Read the model definition and answer for the solid it produces. Units are mm, in the model's axes. Face numbers are marked on the shaded views. A direction names the side the tool comes from. Coordinates: 2 decimals unless noted, no trailing zeros. Write each loop counter-clockwise with the first axis right and the second up, starting at its lowest first coordinate (ties: lowest second). Pieces come first, ordered by that corner, then holes. Notation, with made-up numbers: (51, 44.5) -> (96, 44.5) arc R28 ccw to (96, 63.5) -> close; hole circle Ø11 at (17.5, -38). An arc over 180 degrees is marked (long way). Return JSON: item names as keys, results as strings.
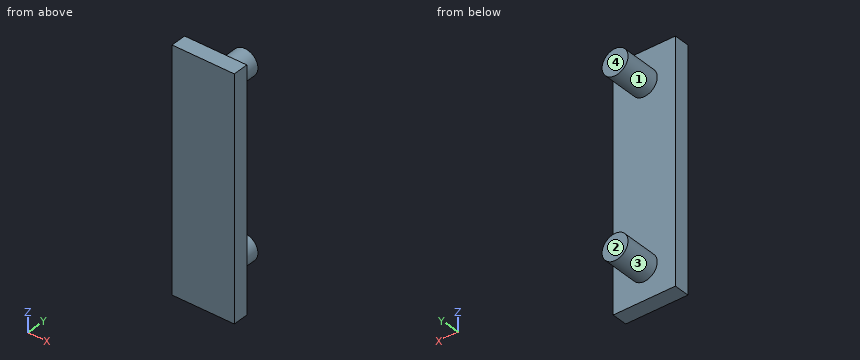
from build123d import *

# Parameters (mm, degrees)
SKETCH3_R             = 2.5
BOSS_EXTRUDE4_DEPTH   = 10
BOSS_EXTRUDE4_2_DEPTH = 10
SKETCH2_W             = 12
SKETCH2_H             = 46
BOSS_EXTRUDE5_DEPTH   = 3


with BuildPart() as part:
    # Sketch3 → Boss-Extrude4 (new body)
    with BuildSketch(Plane(origin=(0, 0, 0), x_dir=(1, 0, 0), z_dir=(0, 1, 0))):
        with Locations((-0.169934853, 17.143306367)):
            Circle(SKETCH3_R)
    extrude(amount=BOSS_EXTRUDE4_DEPTH)



with BuildPart() as body_2:
    # Sketch3 → Boss-Extrude4 2 (new body)
    with BuildSketch(Plane(origin=(0, 0, 0), x_dir=(1, 0, 0), z_dir=(0, 1, 0))):
        with Locations((-0.169934853, -16.856693633)):
            Circle(SKETCH3_R)
    extrude(amount=BOSS_EXTRUDE4_2_DEPTH)


with BuildPart() as part_1:
    add(part.part)

    add(body_2.part)  # Boss-Extrude5 merges body 2
    # Sketch2 → Boss-Extrude5 (add)
    with BuildSketch(Plane(origin=(0, 0, 0), x_dir=(1, 0, 0), z_dir=(0, 1, 0))):
        with Locations((-0.169934853, 0.143306367)):
            Rectangle(SKETCH2_W, SKETCH2_H)
    extrude(amount=BOSS_EXTRUDE5_DEPTH)


solid = part_1.part
1. A tool of negligible diameter and unlimited length cuts with its end or side. For the marked faces 1 and 2, from which of +Z, -Z, +X, -X, +Y, -Y can it reach the whole face along a straight path? Write none if from no direction.
Taken from the geometry:
{"face 1": "+Y", "face 2": "+Z, -Z, +X, -X, +Y"}
2. Consider L1, parallel to Z at x = 0, y = 4.25; L2, parallel to Y at x = 1.75, z = 9.5; L3, parallel to Z at x = 2, y = 6. Determine where each line is inside the solid, lowest interval first.
Taken from the geometry:
{"L1": "z = -19.64 to -14.65, 14.36 to 19.35", "L2": "y = 0 to 3", "L3": "z = -18.38 to -15.9, 15.62 to 18.1"}
3. The part is cut by section C-C (y = 5). Determine the outline of the cut face in (x, z).
Taken from the geometry:
{"outline": "circle Ø5 at (-0.17, -17.14); circle Ø5 at (-0.17, 16.86)"}
4. The part is cut by section A-A (x = -0.25). Determine the outline of the cut face in (y, z).
Taken from the geometry:
{"outline": "(0, -23.14) -> (3, -23.14) -> (3, -19.64) -> (10, -19.64) -> (10, -14.64) -> (3, -14.64) -> (3, 14.36) -> (10, 14.36) -> (10, 19.36) -> (3, 19.36) -> (3, 22.86) -> (0, 22.86) -> close"}
5. The part is cut by section D-D (z = -12.5). Determine the outline of the cut face in (x, y), then the cut area to 3 significant figures.
Taken from the geometry:
{"outline": "(-6.17, 0) -> (5.83, 0) -> (5.83, 3) -> (-6.17, 3) -> close", "area": "36.0 mm2"}
6. The part is cut by section B-B (z = -18). Determine the outline of the cut face in (x, y).
Taken from the geometry:
{"outline": "(-6.17, 0) -> (5.83, 0) -> (5.83, 3) -> (2.18, 3) -> (2.18, 10) -> (-2.52, 10) -> (-2.52, 3) -> (-6.17, 3) -> close"}
7. For a pull along Z with two mould halves and no side action, classify the marked faces 3 and 4 as +Z half, -Z half, draft (parallel to the pull), parting line (faces both ways), or undercut.
Taken from the geometry:
{"face 3": "undercut", "face 4": "draft"}
8. A flat-ended cylindrical pin translates along its axis: pin 1 Ø6 at (x, z) = (-1.5, -3.5) entering from +Y. Find the tip coordinate at first contact, or state that the pin passes through.
Taken from the geometry:
{"pin 1": "stops at y = 3"}
